Here's the drawing with two shaded views (mm, measured from the low corner). I have some questions. Coordinates: 2 decimals unless noted, no trailing zeros. Loops run counter-clockwise (first coordinate to the right, second up) from the corner with the lowest first, then second, coordinate; pieces in that order, holes last.
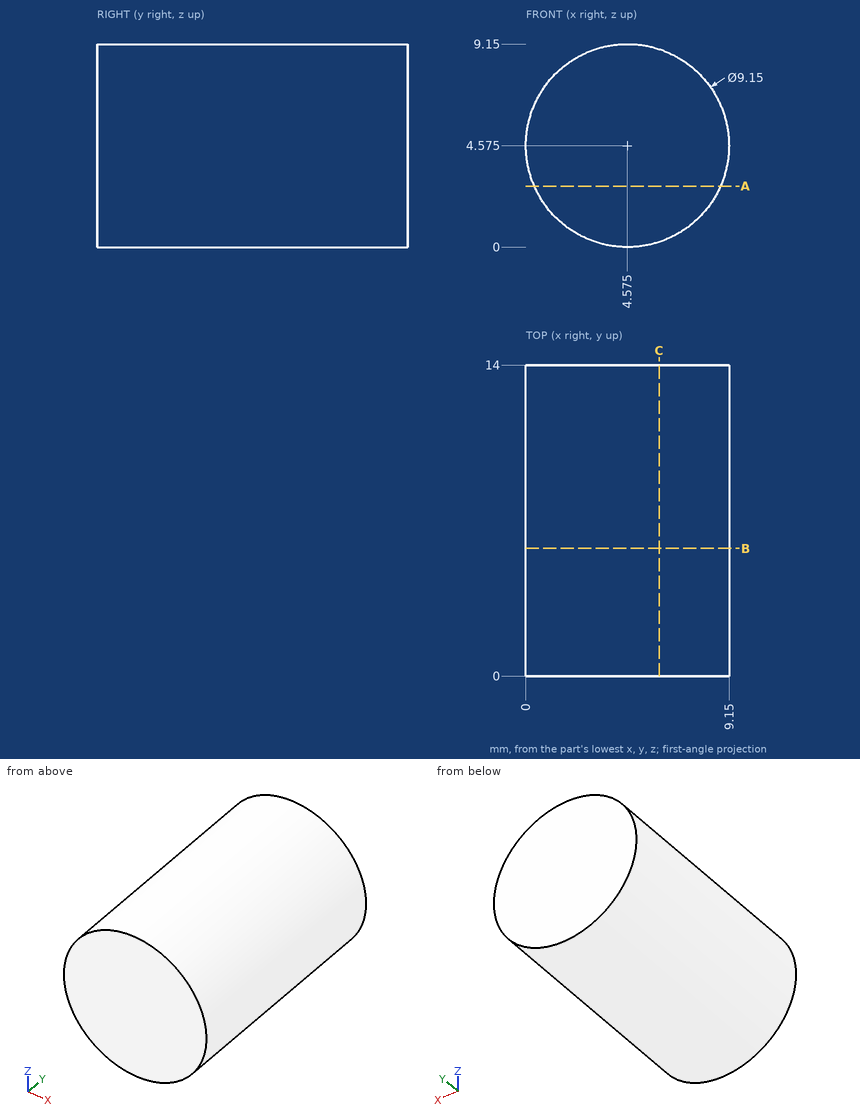
(1) If I drill on probe 1 along X at (y, z) = (11.25, 4.75); probe 2 along X at (y, z) = (6.5, 0.75); probe 3 along Z at (x, y) = (4.25, 11.75), over which ranges is the centre line in solid material (lowest first)?
Check values:
probe 1: x = 0 to 9.15
probe 2: x = 2.07 to 7.08
probe 3: z = 0.01 to 9.14
(2) I want a section at B-B on y = 5.75. Write out the boundary of the cut face in (x, z) (3 decimals).
Check values:
outline: circle Ø9.15 at (4.575, 4.575)
(3) I want a section at C-C on x = 6. Write out the boundary of the cut face in (y, z).
Check values:
outline: (0, 0.23) - (14, 0.23) - (14, 8.92) - (0, 8.92) - close
(4) I want a section at A-A on z = 2.75. Write out the boundary of the cut face in (x, y), then the cut area to 3 significant figures.
Check values:
outline: (0.38, 0) - (8.77, 0) - (8.77, 14) - (0.38, 14) - close
area: 117 mm2
(5) I'm going to push flat-ended pins straight in: pin 1 (1.5 mm diameter, centred on x = 8, y = 1.5, fed in from -Z); pin 2 (1 mm diameter, centred on x = 2, y = 5.5, fed in from -Z); pin 3 (1 mm diameter, centred on x = 3, y = 6.5, fed in from -Z). Where does each tip first touch, or does it pass through?
Check values:
pin 1: stops at z = 0.86
pin 2: stops at z = 0.5
pin 3: stops at z = 0.13
